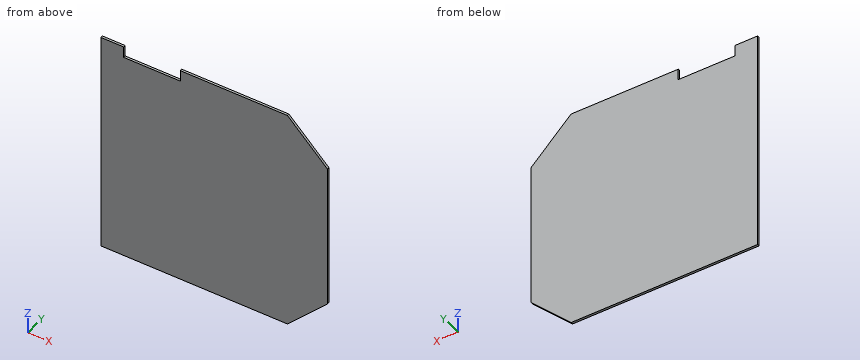
from build123d import *

# Parameters (mm, degrees)
BOSS_EXTRUDE1_DEPTH = 2
SKETCH2_W           = 50
SKETCH2_H           = 10
CUT_EXTRUDE1_DEPTH  = 155.441036988


with BuildPart() as part:
    # Sketch1 → Boss-Extrude1 (new body)
    with BuildSketch(Plane(origin=(0, 0, 0), x_dir=(1, 0, 0), z_dir=(0, 1, 0))):
        Polygon((-82.32233047, 100), (82.32233047, 100), (117.67766953, 64.644660941), (117.67766953, -64.644660941), (82.32233047, -100), (-82.32233047, -100), align=None)
    extrude(amount=BOSS_EXTRUDE1_DEPTH)

    # Sketch2 → Cut-Extrude1 (cut, through all)
    with BuildSketch(Plane(origin=(0, 2, 0), x_dir=(1, 0, 0), z_dir=(0, 1, 0))):
        with Locations((-37.32233047, -95)):
            Rectangle(SKETCH2_W, SKETCH2_H)
    extrude(amount=-CUT_EXTRUDE1_DEPTH, mode=Mode.SUBTRACT)


solid = part.part
Check sheet for the modelled part. Datum: model origin and axes. Units: mm. Round coordinates to 2 decimals unless told otherwise and drop trailing zeros. Order: outer loops, then holes, each group sorted by start corner. A loop starts at its lowest first (then second) coordinate and runs counter-clockwise, first axis right, second up.
(1) Cross-section at C-C, the plane z = -76.5. Enter the section's corners in (x, y), and give its area (3 significant figures).
(2) Go/stop test with a flat-tipped pin: P1, Ø0.6, axis at y = 1.5, z = 92.5, coming from the +X side. Record where the tip stops, or that it passes through.
(3) Cross-section at A-A, the plane y = 1.45. Enter the section's corners in (x, z), and give its area (4 significant figures).
(4) Scan lines: probe 1 along X at (y, z) = (1.5, -82.5); probe 2 along Z at (x, y) = (-58, 1.1); probe 3 along X at (y, z) = (0.35, 89). Record each from-to range of solid material in increasing order.
(5) Cross-section at B-B, the plane x = -40. Enter the section's corners in (y, z).
Check sheet entries:
1. outline: (-82.32, 0) - (105.82, 0) - (105.82, 2) - (-82.32, 2) - close
1. area: 376 mm2
2. P1: stops at x = 90.12
3. outline: (-82.32, -100) - (82.32, -100) - (117.68, -64.64) - (117.68, 64.64) - (82.32, 100) - (-12.32, 100) - (-12.32, 90) - (-62.32, 90) - (-62.32, 100) - (-82.32, 100) - close
3. area: 38,250 mm2
4. probe 1: x = -82.32 to 99.82
4. probe 2: z = -100 to 90
4. probe 3: x = -82.32 to 93.32
5. outline: (0, -100) - (2, -100) - (2, 90) - (0, 90) - close
